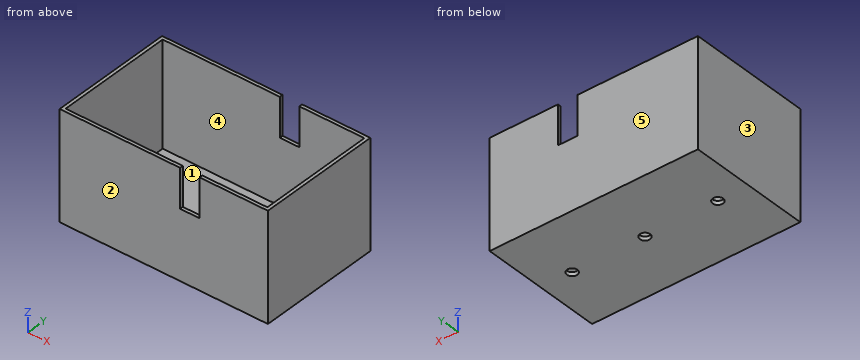
from build123d import *

# Parameters (mm, degrees)
SKETCH_1_W          = 160
SKETCH_1_H          = 95
SKETCH_1_W_2        = 155
SKETCH_1_H_2        = 90
EXTRUDE_1_DEPTH     = 80
SKETCH_3_W          = 160
SKETCH_3_H          = 95
EXTRUDE_2_DEPTH     = 3
SKETCH_4_R          = 4
CUT_EXTRUDE_1_DEPTH = 10
SKETCH_5_W          = 15
SKETCH_5_H          = 30
CUT_EXTRUDE_2_DEPTH = 148.732867027


with BuildPart() as part:
    # ｽｹｯﾁ1 → ﾎﾞｽ - 押し出し1 (new body)
    with BuildSketch(Plane.XY):
        Rectangle(SKETCH_1_W, SKETCH_1_H)
        Rectangle(SKETCH_1_W_2, SKETCH_1_H_2, mode=Mode.SUBTRACT)
    extrude(amount=EXTRUDE_1_DEPTH)

    # ｽｹｯﾁ3 → ﾎﾞｽ - 押し出し2 (add)
    with BuildSketch(Plane(origin=(0, 0, 0), x_dir=(-1, 0, 0), z_dir=(0, 0, -1))):
        Rectangle(SKETCH_3_W, SKETCH_3_H)
    extrude(amount=EXTRUDE_2_DEPTH)

    # ｽｹｯﾁ4 → ｶｯﾄ - 押し出し1 (cut)
    with BuildSketch(Plane.XY):
        Circle(SKETCH_4_R)
        with Locations((-56, 0)):
            Circle(SKETCH_4_R)
        with Locations((56, 0)):
            Circle(SKETCH_4_R)
    extrude(amount=-CUT_EXTRUDE_1_DEPTH, mode=Mode.SUBTRACT)

    # ｽｹｯﾁ5 → ｶｯﾄ - 押し出し2 (cut, through all)
    with BuildSketch(Plane.XZ.offset(47.5)):
        with Locations((20, 65)):
            Rectangle(SKETCH_5_W, SKETCH_5_H)
    extrude(amount=-CUT_EXTRUDE_2_DEPTH, mode=Mode.SUBTRACT)


solid = part.part
Here's how the part is built. I have some questions about the finished solid (model axes, mm). Face numbers are marked on the shaded views. A direction names the side the tool comes from. Coordinates: 2 decimals unless noted, no trailing zeros. Write each loop counter-clockwise with the first axis right and the second up, starting at its lowest first coordinate (ties: lowest second). Pieces come first, ordered by that corner, then holes.
Item 1: I want a section at B-B on x = 56. Write out the boundary of the cut face in (y, z).
Item 2: Will these pins go through, and if not, where does the flat tip stop? pin 1 (5 mm diameter, centred on x = 0, y = 0, fed in from +Z); pin 2 (0.8 mm diameter, centred on x = 17, y = -46, fed in from +Z); pin 3 (8 mm diameter, centred on x = -4.5, y = -32.5, fed in from +Z).
Item 3: On a 3-axis mill with a long thin cutter (end or side, diameter ignored), from which of +Z, -Z, +X, -X, +Y, -Y can I reach the whole of each face in a straight line? I mean the marked faces 1 and 2. Say none if no direction works.
Item 4: I want a section at A-A on z = 53. Write out the boundary of the cut face in (x, y).
Item 5: I want a section at C-C on y = 0. Write out the boundary of the cut face in (x, z), and give its area (3 significant figures).
Item 6: If I drill on line 1 (Y direction, x = -32.5, z = 76); line 2 (Y direction, x = 56, z = -1); line 3 (X direction, y = 21, z = 50), over which ranges is the centre line in solid material (lowest first)?
Item 7: If we mould it in two halves opening along X, with no side actions, what happens to the marked faces 3, 4 and 5? For each: +X half, -X half, draft (parallel to the pull), parting line (faces both ways), or undercut.
Item 8: I want a section at D-D on z = 41. Write out the boundary of the cut face in (x, y).
Findings below:
1. outline: (-47.5, -3) - (-4, -3) - (-4, 0) - (-45, 0) - (-45, 80) - (-47.5, 80) - close; (4, -3) - (47.5, -3) - (47.5, 80) - (45, 80) - (45, 0) - (4, 0) - close
2. pin 1: passes through
2. pin 2: stops at z = 50
2. pin 3: stops at z = 0
3. face 1: +Z
3. face 2: +Z, -Z, +X, -X, -Y
4. outline: (-80, -47.5) - (12.5, -47.5) - (12.5, -45) - (-77.5, -45) - (-77.5, 45) - (12.5, 45) - (12.5, 47.5) - (-80, 47.5) - close; (27.5, -47.5) - (80, -47.5) - (80, 47.5) - (27.5, 47.5) - (27.5, 45) - (77.5, 45) - (77.5, -45) - (27.5, -45) - close
5. outline: (-80, -3) - (-60, -3) - (-60, 0) - (-77.5, 0) - (-77.5, 80) - (-80, 80) - close; (-52, -3) - (-4, -3) - (-4, 0) - (-52, 0) - close; (4, -3) - (52, -3) - (52, 0) - (4, 0) - close; (60, -3) - (80, -3) - (80, 80) - (77.5, 80) - (77.5, 0) - (60, 0) - close
5. area: 808 mm2
6. line 1: y = -47.5 to -45, 45 to 47.5
6. line 2: y = -47.5 to -4, 4 to 47.5
6. line 3: x = -80 to -77.5, 77.5 to 80
7. face 3: -X half
7. face 4: undercut
7. face 5: draft
8. outline: (-80, -47.5) - (80, -47.5) - (80, 47.5) - (-80, 47.5) - close; hole (-77.5, -45) - (77.5, -45) - (77.5, 45) - (-77.5, 45) - close
